Here's how the part is built. I have some questions about the finished solid (model axes, mm). Face numbers are marked on the shaded views. Coordinates: 2 decimals unless noted, no trailing zeros. Write each loop counter-clockwise with the first axis right and the second up, starting at its lowest first coordinate (ties: lowest second). Pieces come first, ordered by that corner, then holes. Notation, with made-up numbers: (-39.75, -35) -> (-5.75, -35) arc R34 ccw to (-5.75, 3) -> close; hole circle Ø10 at (9.25, -7.75). An arc over 180 degrees is marked (long way). Use a Markdown table: item, result. Add a question column.
Item 1: Will these pins go through, and if not, where does the flat tip stop? pin 1 Ø6 at (x, z) = (23, 30) entering from +Y; pin 2 Ø2.5 at (y, z) = (2, 1) entering from +X; pin 3 Ø10 at (x, z) = (39.5, 16) entering from -Y.
Item 2: Imagine slicing it at C-C, the plane x = -36.5. Write out the boundary of the cut face in (y, z).
Item 3: Imagine slicing it at A-A, the plane x = -25. Write out the boundary of the cut face in (y, z), and give its area (3 significant figures).
Item 4: If we mould it in two halves opening along Z, with no side actions, what happens to the marked faces 1 and 2? For each: pulls with the +Z half, pulls with the -Z half, needs draft (parallel to the pull), parting line crosses it, or undercut.
Item 5: If I drill on line 1 along X through (y, z) = (-1, 0); line 2 along Z through (x, y) = (20.5, -0.5); line 3 along Y through (x, z) = (-1.5, -20), over which ranges is the centre line in solid material (lowest first)? Write a range as from..to.
Item 6: Imagine slicing it at B-B, the plane z = 0. Write out the boundary of the cut face in (x, y).
Item 7: Imagine slicing it at D-D, the plane y = -10. Write out the boundary of the cut face in (x, z).
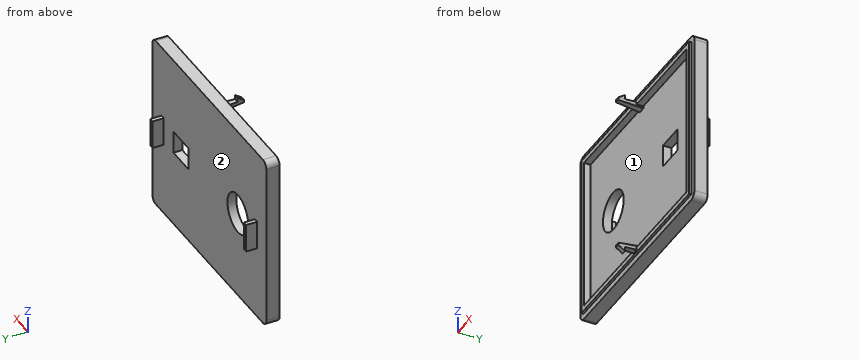
```python
from build123d import *

# Parameters (mm, degrees)
SKETCH1_W           = 100
SKETCH1_H           = 80
BOSS_EXTRUDE1_DEPTH = 7
SKETCH2_W           = 90
SKETCH2_H           = 70
CUT_EXTRUDE1_DEPTH  = 3
SKETCH3_OUTSIDE_W   = 127.65
SKETCH3_OUTSIDE_H   = 107.65
SKETCH3_OUTSIDE_W_2 = 94.6
SKETCH3_OUTSIDE_H_2 = 74.6
CUT_EXTRUDE2_DEPTH  = 1
SKETCH4_W           = 2
SKETCH4_H           = 13
BOSS_EXTRUDE2_DEPTH = 5
SKETCH5_W           = 13
SKETCH5_H           = 10.3
CUT_EXTRUDE3_DEPTH  = 65.412731661
SKETCH6_R           = 9.1
CUT_EXTRUDE4_DEPTH  = 65.412731661
FILLET1_R           = 3
SNAP_START          = -36.217722162
SNAP_HOOK2_DEPTH    = 1.2
SNAP_START_2        = -36.063805806
SNAP_HOOK2_2_DEPTH  = 1.063805806
SNAP_START_3        = -1.403030484
SNAP_HOOK2_3_DEPTH  = 2.314446676
SNAP_START_4        = -1.822292718
SNAP_HOOK2_4_DEPTH  = 3.152971144
SNAP_START_5        = -35
SNAP_HOOK2_5_DEPTH  = 2
SNAP_START_6        = -39
SNAP_HOOK2_6_DEPTH  = 4


with BuildPart() as part:
    # Sketch1 → Boss-Extrude1 (new body)
    with BuildSketch(Plane(origin=(0, 0, 0), x_dir=(1, 0, 0), z_dir=(0, 1, 0))):
        Rectangle(SKETCH1_W, SKETCH1_H)
    extrude(amount=-BOSS_EXTRUDE1_DEPTH)

    # Sketch2 → Cut-Extrude1 (cut)
    with BuildSketch(Plane.XZ.offset(7)):
        Rectangle(SKETCH2_W, SKETCH2_H)
    extrude(amount=-CUT_EXTRUDE1_DEPTH, mode=Mode.SUBTRACT)

    # Sketch3 outside → Cut-Extrude2 (cut)
    with BuildSketch(Plane(origin=(0, -7, 0), x_dir=(-1, 0, 0), z_dir=(0, -1, 0))):
        Rectangle(SKETCH3_OUTSIDE_W, SKETCH3_OUTSIDE_H)
        Rectangle(SKETCH3_OUTSIDE_W_2, SKETCH3_OUTSIDE_H_2, mode=Mode.SUBTRACT)
    extrude(amount=-CUT_EXTRUDE2_DEPTH, mode=Mode.SUBTRACT)

    # Sketch4 → Boss-Extrude2 (add)
    with BuildSketch(Plane(origin=(0, 0, 0), x_dir=(1, 0, 0), z_dir=(0, 1, 0))):
        with Locations((-41, 0)):
            Rectangle(SKETCH4_W, SKETCH4_H)
    boss_extrude2 = extrude(amount=BOSS_EXTRUDE2_DEPTH)

    # Mirror2: Boss-Extrude2 across plane
    add(boss_extrude2.mirror(Plane(origin=(0, 0, 0), x_dir=(0, 0, 1), z_dir=(1, 0, 0))))

    # Sketch5 → Cut-Extrude3 (cut, through all)
    with BuildSketch(Plane(origin=(0, 0, 0), x_dir=(1, 0, 0), z_dir=(0, 1, 0))):
        with Locations((25, 0)):
            Rectangle(SKETCH5_W, SKETCH5_H)
    extrude(amount=-CUT_EXTRUDE3_DEPTH, mode=Mode.SUBTRACT)

    # Sketch6 → Cut-Extrude4 (cut, through all)
    with BuildSketch(Plane(origin=(0, 0, 0), x_dir=(1, 0, 0), z_dir=(0, 1, 0))):
        with Locations(Location((-25, 0, 0), (0, 0, 270))):
            Circle(SKETCH6_R)
    extrude(amount=-CUT_EXTRUDE4_DEPTH, mode=Mode.SUBTRACT)

    # Fillet1
    fillet1_edges = [part.edges().sort_by_distance(p)[0] for p in [
        (50, -3, -40),
        (-50, -3, -40),
        (-50, -3, 40),
        (50, -3, 40),
    ]]
    fillet(fillet1_edges, radius=FILLET1_R)

    # Snap Hook2: read off the stored shape, not the designer's step
    # Snap Hook2 outline → Snap Hook2 (add)
    with BuildSketch(Plane.XY.offset(SNAP_START)):
        Polygon((-1.245807146, -15), (0.754192854, -15), (1.173455088, -7), (-1.66506938, -7), align=None)
    snap_hook2 = extrude(amount=SNAP_HOOK2_DEPTH)

    # Snap Hook2 2 outline → Snap Hook2 2 (add)
    with BuildSketch(Plane.XY.offset(SNAP_START_2)):
        Polygon((-1.66506938, -7), (-1.403030484, -12), (0.911416192, -12), (1.173455088, -7), align=None)
    snap_hook2_2 = extrude(amount=SNAP_HOOK2_2_DEPTH)

    # Snap Hook2 3 outline → Snap Hook2 3 (add)
    with BuildSketch(Plane.YZ.offset(SNAP_START_3)):
        Polygon((-12, -36.217722162), (-15, -36.217722162), (-12, -38.217722162), align=None)
        Polygon((-4, -35), (-4, -33.917722162), (-15, -35.017722162), (-12, -35.017722162), (-12, -35), align=None)
    snap_hook2_3 = extrude(amount=SNAP_HOOK2_3_DEPTH)

    # Snap Hook2 4 outline → Snap Hook2 4 (add)
    with BuildSketch(Plane.YZ.offset(SNAP_START_4)):
        Polygon((-4, -35), (-4, -33.917722162), (-15, -35.017722162), (-12, -35.017722162), (-12, -35), align=None)
    snap_hook2_4 = extrude(amount=SNAP_HOOK2_4_DEPTH)

    # Snap Hook2 5 outline → Snap Hook2 5 (cut)
    with BuildSketch(Plane.XY.offset(SNAP_START_5)):
        Polygon((-1.822292718, -4), (-1.822292718, -16), (-1.193399367, -16), (-1.245807146, -15), align=None)
        Polygon((0.754192854, -15), (0.701785075, -16), (1.330678426, -16), (1.330678426, -4), align=None)
    snap_hook2_5 = extrude(amount=SNAP_HOOK2_5_DEPTH, mode=Mode.SUBTRACT)

    # Snap Hook2 6 outline → Snap Hook2 6 (cut)
    with BuildSketch(Plane.XY.offset(SNAP_START_6)):
        Polygon((-1.822292718, -16), (-1.193399367, -16), (-1.245807146, -15), (-1.403030484, -12), (-1.822292718, -12), align=None)
        Polygon((0.754192854, -15), (0.701785075, -16), (1.330678426, -16), (1.330678426, -12), (0.911416192, -12), align=None)
    snap_hook2_6 = extrude(amount=SNAP_HOOK2_6_DEPTH, mode=Mode.SUBTRACT)

    # Mirror4: Snap Hook2, Snap Hook2 2, Snap Hook2 3, Snap Hook2 4, Snap Hook2 5, Snap Hook2 6 across plane
    add(snap_hook2.mirror(Plane.XY))
    add(snap_hook2_2.mirror(Plane.XY))
    add(snap_hook2_3.mirror(Plane.XY))
    add(snap_hook2_4.mirror(Plane.XY))
    add(snap_hook2_5.mirror(Plane.XY), mode=Mode.SUBTRACT)
    add(snap_hook2_6.mirror(Plane.XY), mode=Mode.SUBTRACT)


solid = part.part
```
Ans:
| question | item | result |
|---|---|---|
| 1 | pin 1 | stops at y = 0 |
| 1 | pin 2 | stops at x = 42 |
| 1 | pin 3 | stops at y = -4 |
| 2 | outline | (-7, -37.3) -> (-6, -37.3) -> (-6, -40) -> (0, -40) -> (0, 40) -> (-6, 40) -> (-6, 37.3) -> (-7, 37.3) -> (-7, 35) -> (-4, 35) -> (-4, -35) -> (-7, -35) -> close |
| 3 | outline | (-7, -37.3) -> (-6, -37.3) -> (-6, -40) -> (0, -40) -> (0, -9.1) -> (-4, -9.1) -> (-4, -35) -> (-7, -35) -> close; (-7, 35) -> (-4, 35) -> (-4, 9.1) -> (0, 9.1) -> (0, 40) -> (-6, 40) -> (-6, 37.3) -> (-7, 37.3) -> close |
| 3 | area | 272 mm^2 |
| 4 | face 1 | undercut |
| 4 | face 2 | needs draft |
| 5 | line 1 | x = -50..-34.1, -15.9..18.5, 31.5..50 |
| 5 | line 2 | z = -40..-5.15, 5.15..40 |
| 5 | line 3 | y = -4..0 |
| 6 | outline | (-50, -6) -> (-47.3, -6) -> (-47.3, -7) -> (-45, -7) -> (-45, -4) -> (-34.1, -4) -> (-34.1, 0) -> (-40, 0) -> (-40, 5) -> (-42, 5) -> (-42, 0) -> (-50, 0) -> close; (-15.9, -4) -> (18.5, -4) -> (18.5, 0) -> (-15.9, 0) -> close; (31.5, -4) -> (45, -4) -> (45, -7) -> (47.3, -7) -> (47.3, -6) -> (50, -6) -> (50, 0) -> (42, 0) -> (42, 5) -> (40, 5) -> (40, 0) -> (31.5, 0) -> close |
| 7 | outline | (-1.51, -36.22) -> (1.02, -36.22) -> (1.02, -34.52) -> (-1.51, -34.52) -> close; (-1.51, 34.52) -> (1.02, 34.52) -> (1.02, 36.22) -> (-1.51, 36.22) -> close |
